Geometry: final body of the model. Coordinates: model frame, mm. A direction names the side the tool comes from. Give positions to 0.01 mm unless a question says otherwise; leave off trailing zeros. Loops run counter-clockwise (first coordinate to the right, second up) from the corner with the lowest first, then second, coordinate; pieces in that order, holes last. Notation, with made-up numbers: (9.25, -11) -> (60.25, -11) arc R32 cw to (60.25, 15) -> close; hole circle Ø2 at (-25.5, 66). An arc over 180 degrees is marked (long way). Answer in a Markdown table with one row per item. Add a question column.
from build123d import *
from OCP.BRepFilletAPI import BRepFilletAPI_MakeFillet

# Parameters (mm, degrees)
SKETCH1_R           = 2.627
BOSS_EXTRUDE1_DEPTH = 6
BOSS_EXTRUDE2_START = -5.08
SKETCH1_3_W         = 38.1
SKETCH1_3_H         = 5.999999938
BOSS_EXTRUDE2_DEPTH = 22.86
SKETCH3_R           = 2.000000064
CUT_EXTRUDE1_DEPTH  = 44.260167546
FILLET1_R1          = 2.54
FILLET1_R2          = 5.08
SKETCH4_R           = 4.2145
SKETCH4_R_2         = 2.627
BOSS_EXTRUDE3_DEPTH = 1.5621
BOSS_EXTRUDE4_START = 8.5979
SKETCH4_2_R         = 4.2145
SKETCH4_2_R_2       = 2.627
BOSS_EXTRUDE4_DEPTH = 1.5621
CHAMFER2_SIZE       = 2.54


with BuildPart() as part:
    # Sketch1 → Boss-Extrude1 (new body)
    with BuildSketch(Plane(origin=(5.08, 0, 0), x_dir=(0, 0, -1), z_dir=(1, 0, 0))):
        Polygon((-19.05, 0), (-19.05, -10.16), (0, -25.4), (19.05, -10.16), (19.05, 0), align=None)
        with Locations((0, -16.51)):
            Circle(SKETCH1_R, mode=Mode.SUBTRACT)
    boss_extrude1 = extrude(amount=BOSS_EXTRUDE1_DEPTH)

    # Sketch1<3> → Boss-Extrude2 (add)
    with BuildSketch(Plane(origin=(5.08, 0, 0), x_dir=(0, 0, -1), z_dir=(1, 0, 0)).offset(BOSS_EXTRUDE2_START)):
        with Locations((0, 2.999999969)):
            Rectangle(SKETCH1_3_W, SKETCH1_3_H)
    boss_extrude2 = extrude(amount=BOSS_EXTRUDE2_DEPTH)

    # Sketch3 → Cut-Extrude1 (cut, through all)
    with BuildSketch(Plane(origin=(0, 5.999999938, 0), x_dir=(1, 0, 0), z_dir=(0, 1, 0))):
        with Locations(Location((17.78, 12.7, 0), (0, 0, 270))):
            Circle(SKETCH3_R)
        with Locations(Location((17.78, -12.7, 0), (0, 0, 90))):
            Circle(SKETCH3_R)
    cut_extrude1 = extrude(amount=-CUT_EXTRUDE1_DEPTH, mode=Mode.SUBTRACT)

    # Mirror2: Boss-Extrude2, Cut-Extrude1 across plane
    add(boss_extrude2.mirror(Plane(origin=(0, 0, 0), x_dir=(0, 0, 1), z_dir=(1, 0, 0))))
    add(cut_extrude1.mirror(Plane(origin=(0, 0, 0), x_dir=(0, 0, 1), z_dir=(1, 0, 0))), mode=Mode.SUBTRACT)

    # Mirror3: Boss-Extrude1 across plane
    add(boss_extrude1.mirror(Plane(origin=(0, 0, 0), x_dir=(0, 0, 1), z_dir=(1, 0, 0))))

    # Fillet1: one fillet with a radius per group of edges: ONE call of the kernel's fillet builder (fillet() takes one radius for all edges)
    fillet1_edges_1 = [part.edges().sort_by_distance(p)[0] for p in [
        (8.08, -10.16, 19.05),
        (8.08, -10.16, -19.05),
        (11.08, 0, 0),
        (22.86, 2.999999969, 19.05),
        (22.86, 2.999999969, -19.05),
        (-22.86, 2.999999969, -19.05),
        (-22.86, 2.999999969, 19.05),
        (-8.08, -10.16, -19.05),
        (-8.08, -10.16, 19.05),
        (-5.08, 0, 0),
        (-11.08, 0, 0),
        (5.08, 0, 0),
    ]]
    fillet1_edges_2 = [part.edges().sort_by_distance(p)[0] for p in [
        (8.08, -25.4, 0),
        (-8.08, -25.4, 0),
    ]]
    fillet1 = BRepFilletAPI_MakeFillet(part.part.solid().wrapped)
    for e in fillet1_edges_1:
        fillet1.Add(FILLET1_R1, e.wrapped)
    for e in fillet1_edges_2:
        fillet1.Add(FILLET1_R2, e.wrapped)
    add(Compound.cast(fillet1.Shape()), mode=Mode.REPLACE)

    # Sketch4 → Boss-Extrude3 (add)
    with BuildSketch(Plane.ZY.offset(-5.08)):
        with Locations(Location((0, -16.51, 0), (0, 0, 180))):
            Circle(SKETCH4_R)
        with Locations((0, -16.51)):
            Circle(SKETCH4_R_2, mode=Mode.SUBTRACT)
    extrude(amount=BOSS_EXTRUDE3_DEPTH)

    # Sketch4<2> → Boss-Extrude4 (add)
    with BuildSketch(Plane.ZY.offset(-5.08).offset(BOSS_EXTRUDE4_START)):
        with Locations(Location((0, -16.51, 0), (0, 0, 180))):
            Circle(SKETCH4_2_R)
        with Locations((0, -16.51)):
            Circle(SKETCH4_2_R_2, mode=Mode.SUBTRACT)
    extrude(amount=BOSS_EXTRUDE4_DEPTH)

    # Chamfer2
    # the kernel refuses this chamfer: 2.54 mm, written as the material it adds along each edge
    with BuildSketch(Plane(origin=(5.08, -16.51, 0), x_dir=(0, 0, -1), z_dir=(0, 1, 0))) as chamfer2_piece_1_section:
        Polygon((4.2145 + CHAMFER2_SIZE, 0), (4.2145, CHAMFER2_SIZE), (4.2145, 0), align=None)
    chamfer2_piece_1 = revolve(axis=Axis((5.08, -16.51, 0), (-1, 0, 0)), mode=Mode.PRIVATE)
    chamfer2_piece_1 = split(chamfer2_piece_1, bisect_by=Plane(origin=(3.5179, -16.51, 5.976913078), z_dir=(1, 0, 0)), keep=Keep.TOP, mode=Mode.PRIVATE)
    add(chamfer2_piece_1)
    with BuildSketch(Plane(origin=(-5.08, -16.51, 0), x_dir=(0, 0, -1), z_dir=(0, 1, 0))) as chamfer2_piece_2_section:
        Polygon((4.2145 + CHAMFER2_SIZE, 0), (4.2145, -CHAMFER2_SIZE), (4.2145, 0), align=None)
    chamfer2_piece_2 = revolve(axis=Axis((-5.08, -16.51, 0), (-1, 0, 0)), mode=Mode.PRIVATE)
    chamfer2_piece_2 = split(chamfer2_piece_2, bisect_by=Plane(origin=(-3.5179, -16.51, 5.976913078), z_dir=(-1, 0, 0)), keep=Keep.TOP, mode=Mode.PRIVATE)
    add(chamfer2_piece_2)


solid = part.part
(1) Material intervals for line 1 along X through (y, z) = (2.85, 12.7); line 2 along Z through (x, y) = (-17.78, 4.4); line 3 along X through (y, z) = (-17, -4.5), sorted ascending. Write a range as from..to.
(2) Cut plane B-B on x = 7.5. Return the cut outline in (y, z), then the cut area to 3 significant figures.
(3) Reachability of faces 1 (the cylindrical face through (19.554, 3.042, 11.777)), 2 (the flat face through (18, 0, 0)), 3 (the flat face through (-18, 0, 0)) from +Z, -Z, +X, -X, +Y, -Y: full face, straight path, thin tool, end or side. Return the list, or none.
(4) Pin query (flat end, axial travel): pin 1 Ø4.5 at (x, z) = (17.78, -12.7) entering from -Y; pin 2 Ø7 at (y, z) = (-16.51, 0) entering from -X; pin 3 Ø6 at (y, z) = (-16.51, 0) entering from +X. Return the tip coordinate at first contact, or that it passes through.
(5) Cut plane C-C on y = -16.51. Return the cut outline in (x, z).
(6) Cut plane D-D on x = -16.5. Return the cut outline in (y, z), then the cut area to 3 significant figures.
(7) Draft query along Y for faces 4 (the flat face through (8, -17, -10.5)), 5 (the flat face through (0, 2, -19.05)), 6 (the flat face through (-5.08, -8, 0)). Return one class per face: +Y half, -Y half, draft (parallel to the pull), parting line (faces both ways), or undercut.
(8) Cut plane A-A on z = -12.7. Return the cut outline in (x, y), then the cut area to 3 significant figures.
Answer list:
| question | item | result |
|---|---|---|
| 1 | line 1 | x = -22.86..-19.78, -15.78..15.78, 19.78..22.86 |
| 1 | line 2 | z = -19.05..-14.7, -10.7..10.7, 14.7..19.05 |
| 1 | line 3 | x = -11.08..-3.52, 3.52..11.08 |
| 2 | outline | (-22.86, -3.17) -> (-10.92, -18.1) arc R2.54 ccw to (-8.94, -19.05) -> (6, -19.05) -> (6, 19.05) -> (-8.94, 19.05) arc R2.54 ccw to (-10.92, 18.1) -> (-22.86, 3.17) arc R5.08 ccw to start; hole circle Ø5.25 at (-16.51, 0) |
| 2 | area | 881 mm² |
| 3 | face 1 | +Y, -Y |
| 3 | face 2 | +Z, -Z, +X, -Y |
| 3 | face 3 | +Z, -Z, -X, -Y |
| 4 | pin 1 | stops at y = 0 |
| 4 | pin 2 | stops at x = -11.08 |
| 4 | pin 3 | stops at x = 11.08 |
| 5 | outline | (-11.08, -11.11) -> (-5.08, -11.11) -> (-5.08, -6.75) -> (-3.52, -5.19) -> (-3.52, -2.63) -> (-11.08, -2.63) -> close; (-11.08, 2.63) -> (-3.52, 2.63) -> (-3.52, 5.19) -> (-5.08, 6.75) -> (-5.08, 11.11) -> (-11.08, 11.11) -> close; (3.52, -5.19) -> (5.08, -6.75) -> (5.08, -11.11) -> (11.08, -11.11) -> (11.08, -2.63) -> (3.52, -2.63) -> close; (3.52, 2.63) -> (11.08, 2.63) -> (11.08, 11.11) -> (5.08, 11.11) -> (5.08, 6.75) -> (3.52, 5.19) -> close |
| 6 | outline | (0, -19.05) -> (6, -19.05) -> (6, -14.24) -> (0, -14.24) -> close; (0, -11.16) -> (6, -11.16) -> (6, 11.16) -> (0, 11.16) -> close; (0, 14.24) -> (6, 14.24) -> (6, 19.05) -> (0, 19.05) -> close |
| 6 | area | 192 mm² |
| 7 | face 4 | -Y half |
| 7 | face 5 | draft |
| 7 | face 6 | undercut |
| 8 | outline | (-22.86, 0) -> (-19.78, 0) -> (-19.78, 6) -> (-22.86, 6) -> close; (-15.78, 0) -> (-13.62, 0) arc R2.54 cw to (-11.08, -2.54) -> (-11.08, -15.24) -> (-5.08, -15.24) -> (-5.08, -2.54) arc R2.54 cw to (-2.54, 0) -> (2.54, 0) arc R2.54 cw to (5.08, -2.54) -> (5.08, -15.24) -> (11.08, -15.24) -> (11.08, -2.54) arc R2.54 cw to (13.62, 0) -> (15.78, 0) -> (15.78, 6) -> (-15.78, 6) -> close; (19.78, 0) -> (22.86, 0) -> (22.86, 6) -> (19.78, 6) -> close |
| 8 | area | 415 mm² |
